Could you check a few things on this model? Use its own coordinates, in mm. Coordinates: 2 decimals unless noted, no trailing zeros. Order: outer loops, then holes, each group sorted by start corner. A loop starts at its lowest first (then second) coordinate and runs counter-clockwise, first axis right, second up. Notation, with made-up numbers: (20, 65) -> (24, 65) arc R17 cw to (24, 95) -> close; hole circle Ø11 at (42, -12). An arc over 180 degrees is marked (long way). Put each result on its own line as item: value. Start each with the question number.
Q1. If we section it at A-A (x = 86): Please give me the cut outline in (y, z), and give its area (4 significant figures).
Q2. Will these pins go through, and if not, where does the flat tip stop? pin 1 (1.5 mm diameter, centred on x = 165, y = 31.5, fed in from -Z); pin 2 (3 mm diameter, centred on x = 190.8, y = 15, fed in from +Z); pin 3 (5 mm diameter, centred on x = 157.5, y = 51.5, fed in from +Z).
Q3. If we section it at B-B (z = 1): Count the separate pieces of the cut face and the enclosed holes in it, and give its area (3 significant figures).
Q4. Please list where these lines run through material, in increasing order: line 1 along Y through (x, z) = (190.8, 1.3); line 2 along X through (y, z) = (29.5, 1.1); line 3 along X through (y, z) = (36, 0.25).
from build123d import *

# Parameters (mm, degrees)
SKETCH_W        = 198
SKETCH_H        = 58
PAD_DEPTH       = 1.65
SKETCH001_R     = 6.1
SKETCH001_R_2   = 1.75
SKETCH001_R_3   = 1.5
SKETCH001_W     = 18
SKETCH001_H     = 32
SKETCH001_W_2   = 20
SKETCH001_H_2   = 7
POCKET_DEPTH    = 5
SKETCH002_W     = 3
SKETCH002_H     = 20.3
SKETCH002_H_2   = 24
POCKET001_DEPTH = 0.5


with BuildPart() as part:
    # Sketch → Pad (new body)
    with BuildSketch(Plane.XY):
        with Locations((99, 29)):
            Rectangle(SKETCH_W, SKETCH_H)
    extrude(amount=PAD_DEPTH)

    # Sketch001 (on Face6 of Pad) → Pocket (cut)
    with BuildSketch(Plane.XY.offset(1.65)):
        with Locations((14.95, 43.825)):
            Circle(SKETCH001_R)
        with Locations((164.8, 43)):
            Circle(SKETCH001_R_2)
        with Locations((190.8, 43)):
            Circle(SKETCH001_R_2)
        with Locations((164.8, 15)):
            Circle(SKETCH001_R_2)
        with Locations((190.8, 15)):
            Circle(SKETCH001_R_2)
        with Locations((77.5, 51.5)):
            Circle(SKETCH001_R_3)
        with Locations((77.5, 6.5)):
            Circle(SKETCH001_R_3)
        with Locations((157.5, 6.5)):
            Circle(SKETCH001_R_3)
        with Locations((157.5, 51.5)):
            Circle(SKETCH001_R_3)
        with Locations((177.8, 29)):
            Rectangle(SKETCH001_W, SKETCH001_H)
        with Locations((45.49, 24.925)):
            Rectangle(SKETCH001_W_2, SKETCH001_H_2)
        Polygon((80, 51.5), (155, 51.5), (155, 6.5), (136, 6.5), (136, 5.5), (99, 5.5), (99, 6.5), (80, 6.5), align=None)
    extrude(amount=-POCKET_DEPTH, mode=Mode.SUBTRACT)

    # Sketch002 → Pocket001 (cut)
    with BuildSketch(Plane.XY):
        with Locations((77.5, 29.15)):
            Rectangle(SKETCH002_W, SKETCH002_H)
        with Locations((164.8, 29)):
            Rectangle(SKETCH002_W, SKETCH002_H_2)
    extrude(amount=POCKET001_DEPTH, mode=Mode.SUBTRACT)


solid = part.part
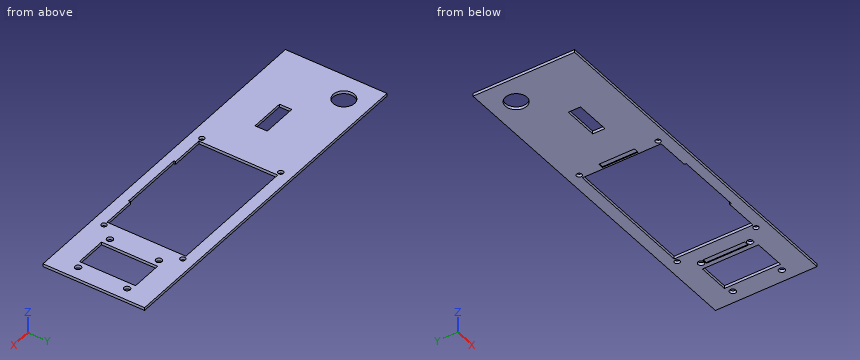
The answers:
1. outline: (0, 0) -> (6.5, 0) -> (6.5, 1.65) -> (0, 1.65) -> close; (51.5, 0) -> (58, 0) -> (58, 1.65) -> (51.5, 1.65) -> close
1. area: 21.45 mm^2
2. pin 1: z = 0.5
2. pin 2: through
2. pin 3: z = 1.65
3. separate pieces: 1
3. enclosed holes: 12
3. area: 7,170 mm^2
4. line 1: 0 to 13.25, 16.75 to 41.25, 44.75 to 58
4. line 2: 0 to 80, 155 to 168.8, 186.8 to 198
4. line 3: 0 to 76, 79 to 80, 155 to 163.3, 166.3 to 168.8, 186.8 to 198
